Work out the finished part from the listing and answer in its coordinate system (mm). Round coordinates to 2 decimals unless told otherwise and drop trailing zeros. Order: outer loops, then holes, each group sorted by start corner. A loop starts at its lowest first (then second) coordinate and runs counter-clockwise, first axis right, second up. Notation, with made-up numbers: (-15, 28) - (8, 28) arc R17 cw to (8, 41) - close; hole circle Ø1 at (14, 16). An arc over 180 degrees is marked (long way). Use CSV: the item, a comma, the result in double quotes.
Autodesk Fusion 360 part; units mm, degrees
sketch "Boceto1" plane through (0, 0, 0) normal (0, 0, 1) x (1, 0, 0)
  circle A0 centre (0, 0) radius 30
  circle A1 centre (200, 0) radius 20
  line L0 (-0.0033, 30) -> (200.9963, 19.9752)
  line L1 (200.9963, -19.9752) -> (-0.0033, -30)
  circle A2 centre (0, 0) radius 5
  circle A3 centre (200, 0) radius 5
extrude "Extruir1" add sketch "Boceto1" along normal blind 4 contours A0 L0 L1 | A0 A1 L0 L1 | A1
sketch "Boceto2" plane through (0, 0, 4) normal (0, 0, 1) x (-1, 0, 0)
  circle A0 centre (-200, 0) radius 5
  circle A1 centre (0, 0) radius 5
  arc A2 (0.0033, -30) -> (0.0033, 30) centre (0, 0) ccw
  line L0 (0.0033, 30) -> (-200.9963, 19.9752)
  arc A3 (-200.9963, 19.9752) -> (-200.9963, -19.9752) centre (-200, 0) ccw
  line L1 (-200.9963, -19.9752) -> (0.0033, -30)
  line L2 (0, 0) -> (-40, 0)
  line L3 (-40, 0) -> (-80, 0)
  line L4 (-80, 0) -> (-120, 0)
  line L5 (-120, 0) -> (-160, 0)
  line L6 (-160, 0) -> (-200, 0)
  line L7 (0, 0) -> (15, 0)
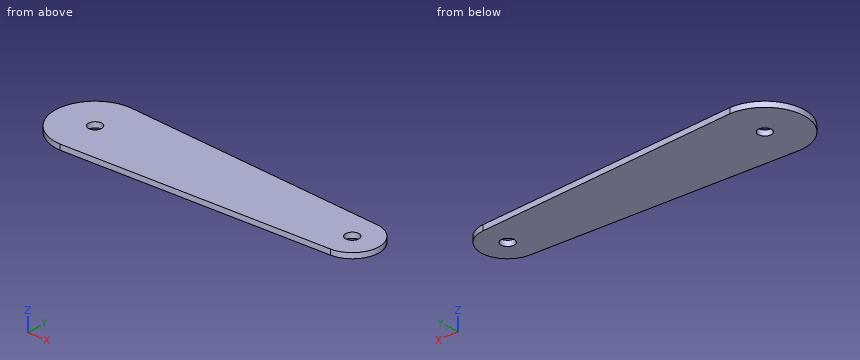
(1) Find section B-B (x = 198.5). Determine the outline of the cut face in (y, z), and give its area (3 significant figures).
Findings below:
outline,"(-20.1, 0) - (-4.77, 0) - (-4.77, 4) - (-20.1, 4) - close; (4.77, 0) - (20.1, 0) - (20.1, 4) - (4.77, 4) - close"
area,"123 mm²"
(2) Find section A-A (y = 0). Determine the outline of the cut face in (x, z), and give its area (3 significant figures).
Findings below:
outline,"(-30, 0) - (-5, 0) - (-5, 4) - (-30, 4) - close; (5, 0) - (195, 0) - (195, 4) - (5, 4) - close; (205, 0) - (220, 0) - (220, 4) - (205, 4) - close"
area,"920 mm²"
(3) Find section D-D (x = 97.5). Determine the outline of the cut face in (y, z).
Findings below:
outline,"(-25.14, 0) - (25.14, 0) - (25.14, 4) - (-25.14, 4) - close"
(4) Each of these flat-tipped pins is pushed along its axis until it touches: pin 1 (1 mm diameter, centred on y = -12, z = 3.5, fed in from -X); pin 2 (1 mm diameter, centred on x = 12, y = 7.5, fed in from -Z); pin 3 (1 mm diameter, centred on x = 157.5, z = 3, fed in from -Y). Where does it stop, or does it pass through?
Findings below:
pin 1,"stops at x = -27.71"
pin 2,"stops at z = 0"
pin 3,"stops at y = -22.17"
(5) Find section C-C (z = 3.15). Determine the outline of the cut face in (x, y).
Findings below:
outline,"(0, -30) - (201, -19.98) arc R20 ccw to (201, 19.98) - (0, 30) arc R30 ccw to start; hole circle Ø10 at (0, 0); hole circle Ø10 at (200, 0)"
(6) Find the intervals of material crossed by L1, parallel to X at y = -0.5, z = 3.5; L2, parallel to Y at x = 200, z = 2.15; L3, parallel to Y at x = 0, z = 3, in increasing order. Write a range as from..to.
Findings below:
L1,"x = -30..-4.97, 4.97..195.03, 204.97..219.99"
L2,"y = -20.02..-5, 5..20.02"
L3,"y = -30..-5, 5..30"
